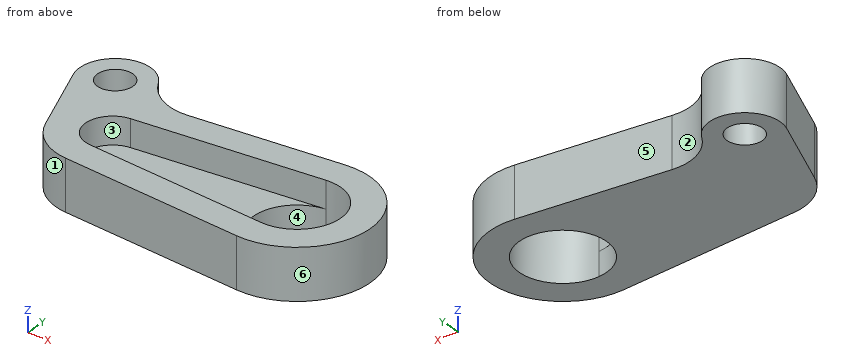
Autodesk Inventor part; units mm, degrees
ref_plane "Work Plane1" through (3.5948, -3.4691, -4.3) normal (0, 0, -1) x (0, 1, 0)
ref_plane "YZ Plane" through (0, 0, 0) normal (1, 0, 0) x (0, 1, 0)
ref_plane "XZ Plane" through (0, 0, 0) normal (0, 1, 0) x (-1, 0, 0)
sketch "Sketch1" plane through (0, 0, 0) normal (0, 0, 1) x (1, 0, 0)
  line L0 (6.7664, -3.387) -> (-9.1111, -1.9923)
  line L1 (6.7664, 3.387) -> (-9.1111, 1.9923)
  arc A0 (-9.1111, 1.9923) -> (-9.1111, -1.9923) centre (-8.9361, 0) ccw
  circle A1 centre (-5.2361, 0) radius 0.5
  circle A2 centre (-7.1361, 0) radius 0.5
  circle A3 centre (-9.0361, 0) radius 0.5
  circle A4 centre (2.3639, 0) radius 0.5
  circle A5 centre (0.4639, 0) radius 0.5
  circle A6 centre (-1.4361, 0) radius 0.5
  circle A7 centre (-3.3361, 0) radius 0.5
  arc A8 (6.7664, -3.387) -> (6.7664, 3.387) centre (7.0639, 0) ccw
  line L2 (-9.1373, 2.2912) -> (6.7402, 3.6858)
  arc A9 (6.7402, -3.6858) -> (6.7402, 3.6858) centre (7.0639, 0) ccw
  line L3 (6.7402, -3.6858) -> (-9.1373, -2.2912)
  arc A10 (-9.1373, 2.2912) -> (-9.1373, -2.2912) centre (-8.9361, 0) ccw
  line L4 (6.5214, 6.1762) -> (-9.3561, 4.7816)
  arc A11 (-9.3561, 4.7816) -> (-9.3561, -4.7816) centre (-8.9361, 0) ccw
  line L5 (-9.3561, -4.7816) -> (6.5214, -6.1762)
  arc A12 (6.5214, -6.1762) -> (6.5214, 6.1762) centre (7.0639, 0) ccw
  point P0 (0, 0)
  dimension "d0" = 0.3
  dimension "d1" = 2.5
ref_plane "Work Plane1" through (3.5948, -3.4691, -4.3) normal (0, 0, -1) x (0, 1, 0)
extrude "Extrusion1" add sketch "Sketch1" against normal up to surface (4.3 mm away) contours A12 L5 A11 L4
sketch "Sketch2" plane through (7.0639, 0, -4.3) normal (0, 0, -1) x (-1, 0, 0)
  line L0 (0.3238, -3.6858) -> (16.2013, -2.2912)
  arc A0 (16.2013, -2.2912) -> (16.2012, 2.2912) centre (16, 0) ccw
  line L1 (16.2012, 2.2912) -> (0.3237, 3.6858)
  arc A1 (0.2975, -3.387) -> (0.2975, 3.387) centre (0, 0) ccw
  circle A2 centre (0, 0) radius 3.7
  point P0 (7.0639, 0)
  point P1 (0.3237, 3.6858)
extrude "Extrusion2" add sketch "Sketch2" against normal blind 2 contours A2 L1 A0 L0
sketch "Sketch6" plane through (0, 0, 0) normal (0, 0, 1) x (1, 0, 0)
  circle A0 centre (-13.2269, 5.8971) radius 0.5
  circle A1 centre (-13.2269, 5.8971) radius 1.5
  arc A2 (-9.3561, 4.7816) -> (-9.3561, -4.7816) centre (-8.9361, 0) ccw
  line L0 (6.5214, 6.1762) -> (-9.3561, 4.7816)
  circle A3 centre (-13.2269, 5.8971) radius 3
  line L1 (-16.0133, 4.7853) -> (-13.3943, -1.7788)
  arc A4 (-10.6035, 7.3522) -> (-6.2746, 5.0523) centre (-6.6683, 9.535) ccw
  point P0 (0, 0)
  dimension "d10" = 3
  dimension "d11" = 6
  dimension "d12" = 9
extrude "Extrusion5" add sketch "Sketch6" against normal up to surface (4.3 mm away) contours A2 A3 A4 L0 | A2 A3 | A2 L1 A3 picked at (-12.6304, 3.6481)
properties part number "GripperLeft_3DPrint"
Source: CAD feature listing. Evaluate the final solid. Frame: model axes, mm. Face numbers are marked on the shaded views. A direction names the side the tool comes from. Give positions to 0.01 mm unless a question says otherwise; leave off trailing zeros. Write each loop counter-clockwise with the first axis right and the second up, starting at its lowest first coordinate (ties: lowest second). Pieces come first, ordered by that corner, then holes.
1. Section query B-B (y = 0). Return the cut outline in (x, z), then the cut area to 3 significant figures.
2. Section query D-D (x = 0.75). Return the cut outline in (y, z).
3. First-contact query: pin 1 (6 mm diameter, centred on x = 9, y = -3.5, fed in from +Z); pin 2 (6 mm diameter, centred on x = 7.06, y = 0, fed in from -Z); pin 3 (3.5 mm diameter, centred on x = -6.5, y = -0.5, fed in from +Z). Flat tips, straight axial feed; report the tip coordinate or a pass-through.
4. Section query C-C (z = -2.8). Return the cut outline in (x, y), then the cut area to 3 significant figures.
5. Pull-direction query (Y, two-part tool) for the marked faces 4, 5 and 6; classes: +Y half, -Y half, draft (parallel to the pull), parting line (faces both ways), or undercut.
6. Access query for the marked faces 1, 2 and 3. Directions: +Z, -Z, +X, -X, +Y, -Y. A direction counts if a zero-diameter tool reaches every point of the face in a straight line with its end or side. Return the directions, or none.
7. Section query A-A (x = 7.75). Return the cut outline in (y, z).
8. Material intervals for line 1 along X through (y, z) = (1.5, -1.3); line 2 along Y through (x, z) = (8, -0.2); line 3 along Y through (x, z) = (0.25, -1.2), sorted ascending.
Output values:
1. outline: (-14.1, -4.3) - (3.36, -4.3) - (3.36, -2.3) - (-11.24, -2.3) - (-11.24, 0) - (-14.1, 0) - close; (10.76, -4.3) - (13.26, -4.3) - (13.26, 0) - (10.76, 0) - close
1. area: 52.3 mm2
2. outline: (-5.67, -4.3) - (5.67, -4.3) - (5.67, 0) - (3.16, 0) - (3.16, -2.3) - (-3.16, -2.3) - (-3.16, 0) - (-5.67, 0) - close
3. pin 1: stops at z = 0
3. pin 2: passes through
3. pin 3: stops at z = -2.3
4. outline: (-16.01, 4.79) - (-13.39, -1.78) arc R4.8 ccw to (-9.36, -4.78) - (6.52, -6.18) arc R6.2 ccw (long way) to (6.52, 6.18) - (-6.27, 5.05) arc R4.5 cw to (-10.6, 7.35) arc R3 ccw to start; hole circle Ø3 at (-13.23, 5.9); hole circle Ø7.4 at (7.06, 0)
4. area: 258 mm2
5. face 4: undercut
5. face 5: +Y half
5. face 6: parting line
6. face 1: +Z, -Z, -X, -Y
6. face 2: +Z, -Z, +Y
6. face 3: +Z
7. outline: (-6.16, -4.3) - (-3.64, -4.3) - (-3.64, 0) - (-6.16, 0) - close; (3.64, -4.3) - (6.16, -4.3) - (6.16, 0) - (3.64, 0) - close
8. line 1: x = -14.7 to -10.68, 10.45 to 13.08
8. line 2: y = -6.13 to -3.58, 3.58 to 6.13
8. line 3: y = -5.63 to -3.12, 3.12 to 5.63
